Can you work these out from the model? Positions are in its coordinate system, mm. Coordinates: 2 decimals unless noted, no trailing zeros. Order: outer loops, then holes, each group sorted by start corner. A loop starts at its lowest first (then second) coordinate and runs counter-clockwise, first axis right, second up. Notation, with made-up numbers: (55.25, 82.5) -> (104.25, 82.5) arc R19 ccw to (104.25, 111.5) -> close; hole circle Ø3 at (16.25, 8). An arc over 180 degrees is marked (long way). Use a Markdown table: item, result. Add a question column.
1. Suppose I cut it at A-A, the plane z = 0. List the corners of the cut face in (x, y) for me, then the cut area to 3 significant figures.
2. For pin 1 Ø1.6 at (x, y) = (-2.5, 0.5) entering from -Z; pin 2 Ø1.5 at (x, y) = (7.5, 4) entering from +Z; pin 3 Ø3 at (x, z) = (-3, -1.5) entering from +Y, each with a flat end and sliding along its axis, tell me the tip position at first contact or that it passes through.
3. We'd pull the mould along Z, two halves only. Please class faces 1 (the flat face through (0, 2, 0)), 2 (the cylindrical face through (0.098, 2.301, -4.215)), 3 (the flat face through (-0.2, 0.8, -5)), 4 (the cylindrical face through (6, 1, 0)): pulls with the +Z half, pulls with the -Z half, needs draft (parallel to the pull), parting line crosses it, or undercut.
4. Suppose I cut it at D-D, the plane x = 7.5. List the corners of the cut face in (y, z) for me.
5. If I drill on line 1 along X through (y, z) = (1.2, 0); line 2 along X through (y, z) = (0.35, 1); line 3 along Z through (x, y) = (-3.5, 0.4), over which ranges is the centre line in solid material (lowest first)? Write a range as from..to.
6. Suppose I cut it at C-C, the plane y = 0.6. List the corners of the cut face in (x, z) for me, then the cut area to 3 significant figures.
```python
from build123d import *

# Parameters (mm, degrees)
SKETCH2_W           = 22
SKETCH2_H           = 10
SKETCH2_R           = 1.5
BOSS_EXTRUDE1_DEPTH = 2
SKETCH3_W           = 3
SKETCH3_H           = 3
SKETCH3_R           = 1
BOSS_EXTRUDE2_DEPTH = 7
FILLET1_R           = 1.5
FILLET2_R           = 1
FILLET3_R           = 1.5


with BuildPart() as part:
    # Sketch2 → Boss-Extrude1 (new body)
    with BuildSketch(Plane(origin=(0, 0, 0), x_dir=(1, 0, 0), z_dir=(0, 1, 0))):
        Rectangle(SKETCH2_W, SKETCH2_H)
        with Locations(Location((-7.5, 0, 0), (0, 0, 270))):
            Circle(SKETCH2_R, mode=Mode.SUBTRACT)
        with Locations(Location((7.5, 0, 0), (0, 0, 270))):
            Circle(SKETCH2_R, mode=Mode.SUBTRACT)
    extrude(amount=BOSS_EXTRUDE1_DEPTH)

    # Sketch3 → Boss-Extrude2 (add, symmetric)
    with BuildSketch(Plane(origin=(0, 0, 0), x_dir=(0, 0, -1), z_dir=(1, 0, 0))):
        with Locations((6, 3.5)):
            Rectangle(SKETCH3_W, SKETCH3_H)
        with Locations((6, 3.5)):
            Circle(SKETCH3_R, mode=Mode.SUBTRACT)
    extrude(amount=BOSS_EXTRUDE2_DEPTH, both=True)

    # Fillet1
    fillet1_edges = [part.edges().sort_by_distance(p)[0] for p in [
        (0, 5, -4.5),
        (0, 5, -7.5),
    ]]
    fillet(fillet1_edges, radius=FILLET1_R - 0.0001)  # a hair under: the kernel refuses the full size

    # Fillet2
    fillet2_edges = [part.edges().sort_by_distance(p)[0] for p in [
        (0, 2, -5),
        (0, 2, -4.5),
    ]]
    fillet(fillet2_edges, radius=FILLET2_R)

    # Fillet3
    fillet3_edges = [part.edges().sort_by_distance(p)[0] for p in [
        (0, 2, -7.5),
    ]]
    fillet(fillet3_edges, radius=FILLET3_R - 0.0001)  # a hair under: the kernel refuses the full size


solid = part.part
```
Worked out:
| question | item | result |
|---|---|---|
| 1 | outline | (-11, 0) -> (-9, 0) -> (-9, 2) -> (-11, 2) -> close; (-6, 0) -> (6, 0) -> (6, 2) -> (-6, 2) -> close; (9, 0) -> (11, 0) -> (11, 2) -> (9, 2) -> close |
| 1 | area | 32.0 mm² |
| 2 | pin 1 | stops at z = -5.05 |
| 2 | pin 2 | stops at z = -4.5 |
| 2 | pin 3 | stops at y = 2 |
| 3 | face 1 | needs draft |
| 3 | face 2 | pulls with the +Z half |
| 3 | face 3 | pulls with the -Z half |
| 3 | face 4 | undercut |
| 4 | outline | (0, -5) -> (2, -5) -> (2, -1.5) -> (0, -1.5) -> close; (0, 1.5) -> (2, 1.5) -> (2, 5) -> (0, 5) -> close |
| 5 | line 1 | x = -11..-9, -6..6, 9..11 |
| 5 | line 2 | x = -11..-8.62, -6.38..6.38, 8.62..11 |
| 5 | line 3 | z = -5..5 |
| 6 | outline | (-11, -5) -> (11, -5) -> (11, 5) -> (-11, 5) -> close; hole circle Ø3 at (-7.5, 0); hole circle Ø3 at (7.5, 0) |
| 6 | area | 206 mm² |
